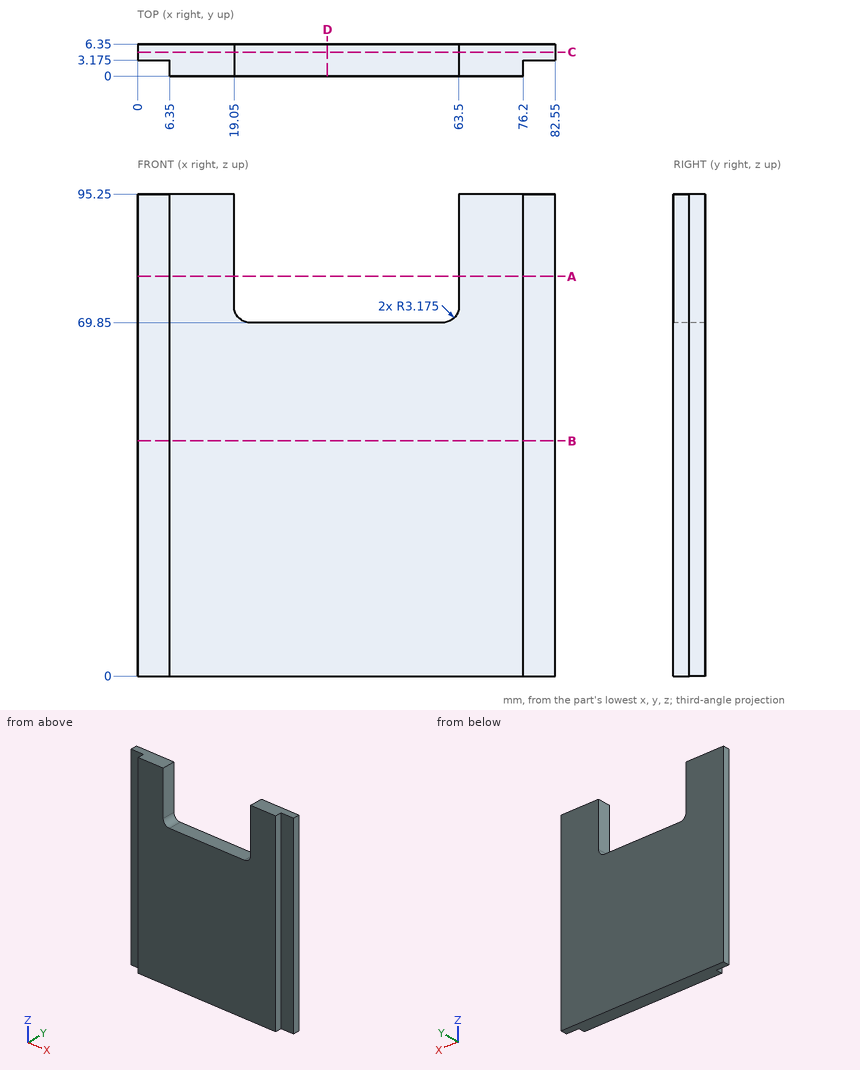
The figure shows three views and two pictorial views of one solid part (mm, origin at its lowest corner). Answer the questions. Round coordinates to 2 decimals unless told otherwise and drop trailing zeros. Order: outer loops, then holes, each group sorted by start corner. A loop starts at its lowest first (then second) coordinate and runs counter-clockwise, first axis right, second up.
Q1. A cutting plane is placed at D-D, the plane x = 37.5. Determine the outline of the cut face in (y, z).
Solution:
outline: (0, 0) - (6.35, 0) - (6.35, 69.85) - (0, 69.85) - close
Q2. A cutting plane is placed at A-A, the plane z = 79. Determine the outline of the cut face in (x, y) (3 decimals).
Solution:
outline: (0, 3.175) - (6.35, 3.175) - (6.35, 0) - (19.05, 0) - (19.05, 6.35) - (0, 6.35) - close; (63.5, 0) - (76.2, 0) - (76.2, 3.175) - (82.55, 3.175) - (82.55, 6.35) - (63.5, 6.35) - close
Q3. A cutting plane is placed at C-C, the plane y = 4.75. Determine the outline of the cut face in (x, z) (3 decimals).
Solution:
outline: (0, 0) - (82.55, 0) - (82.55, 95.25) - (63.5, 95.25) - (63.5, 73.025) arc R3.175 cw to (60.325, 69.85) - (22.225, 69.85) arc R3.175 cw to (19.05, 73.025) - (19.05, 95.25) - (0, 95.25) - close
Q4. Given pin 1 Ø1 at (y, z) = (1.5, 60) entering from -X; pin 2 Ø12 at (x, z) = (49, 75.5) entering from -Y; pin 3 Ø5 at (x, z) = (80.5, 38.5) entering from -Y (3 decimals); pin 4 Ø1.9 at (x, y) = (50.5, 4.5) entering from +Z, each flat-ended and moving along its own axis, determine where each tip first touches the part or whether it passes through.
Solution:
pin 1: stops at x = 6.35
pin 2: stops at y = 0
pin 3: stops at y = 3.175
pin 4: stops at z = 69.85
Q5. Find the intervals of material crossed by line 1 along Z through (x, y) = (40.5, 4.5); line 2 along X through (y, z) = (0.5, 83); line 3 along X through (y, z) = (3.5, 71), in increasing order.
Solution:
line 1: z = 0 to 69.85
line 2: x = 6.35 to 19.05, 63.5 to 76.2
line 3: x = 0 to 19.78, 62.77 to 82.55
Q6. A cutting plane is placed at B-B, the plane z = 46.5. Determine the outline of the cut face in (x, y) (3 decimals).
Solution:
outline: (0, 3.175) - (6.35, 3.175) - (6.35, 0) - (76.2, 0) - (76.2, 3.175) - (82.55, 3.175) - (82.55, 6.35) - (0, 6.35) - close
